Autodesk Inventor part; units mm, degrees
ref_plane "YZ Plane" through (0, 0, 0) normal (1, 0, 0) x (0, 1, 0)
ref_plane "XZ Plane" through (0, 0, 0) normal (0, 1, 0) x (-1, 0, 0)
ref_plane "XY Plane" through (0, 0, 0) normal (0, 0, 1) x (1, 0, 0)
sketch "Skizze1" plane through (0, 0, 0) normal (0, 1, 0) x (-1, 0, 0)
  line L0 (0, 0) -> (10, 0)
  line L1 (10, 0) -> (10, -30)
  line L2 (10, -30) -> (0, -30)
  line L3 (0, -30) -> (0, 0)
  dimension "d0" = 10
  dimension "d1" = 30
extrude "Extrusion1" add sketch "Skizze1" along normal blind 30
sketch "Skizze2" plane through (0, 30, 0) normal (0, 1, 0) x (1, 0, 0)
  line L0 (-10, 0) -> (0, 0)
  line L1 (0, 0) -> (0, 30)
  point P0 (-5, 4.75)
  point P1 (-5, 25.25)
  dimension "d4" = 20.5
  dimension "d5" = 4.75
  dimension "d6" = 5
hole "Bohrung1" at (-5, 30, -4.75) at (-5, 30, -25.25) direction (0, -1, 0) diameter 2 depth 10 tip angle 118
sketch "Skizze4" plane through (0, 0, 0) normal (0, -1, 0) x (1, 0, 0)
  line L0 (0, 0) -> (-10, 0)
  line L1 (0, -30) -> (0, 0)
  point P0 (-5, -22.5)
  point P1 (-5, -7.5)
  dimension "d21" = 15
  dimension "d22" = 7.5
  dimension "d23" = 5
hole "Bohrung3" at (-5, 0, -22.5) at (-5, 0, -7.5) direction (0, 1, 0) diameter 2.5 depth 10 tip angle 118
properties part number "KugelRadStützen"
Input: part model. Units: mm. Frame: model coordinates. A direction names the side the tool comes from. Give positions to 0.01 mm unless a question says otherwise; leave off trailing zeros. Order: outer loops, then holes, each group sorted by start corner. A loop starts at its lowest first (then second) coordinate and runs counter-clockwise, first axis right, second up.
1. Pin query (flat end, axial travel): pin 1 (1.5 mm diameter, centred on x = -5, z = -7.5, fed in from -Y). Return the tip coordinate at first contact, or that it passes through.
Derived:
pin 1: stops at y = 10.3
2. Material intervals for L1, parallel to X at y = 25, z = -4.75, sorted ascending.
Derived:
L1: x = -10 to -6, -4 to 0
3. Reachability of faces 4 (the flat face through (-5, 0, -15)), 5 (the cylindrical face through (-4.521, 5.07, -23.655)), 6 (the cylindrical face through (-5.676, 24.93, -25.987)) from +Z, -Z, +X, -X, +Y, -Y: full face, straight path, thin tool, end or side. Return the list, or none.
Derived:
face 4: +Z, -Z, +X, -X, -Y
face 5: -Y
face 6: +Y
4. Mould query, pull axis Z, two halves, no side actions, for faces 1 (the cylindrical face through (-4.24, 5.07, -6.51)), 2 (the flat face through (-5, 15, 0)), 3 (the flat face through (-5, 15, -30)). Classes: released by +Z, released by -Z, zero draft, split by the parting line, or undercut.
Derived:
face 1: undercut
face 2: released by +Z
face 3: released by -Z
5. Section B-B on y = 5. Return the cut outline in (x, z).
Derived:
outline: (-10, -30) - (0, -30) - (0, 0) - (-10, 0) - close; hole circle Ø2.5 at (-5, -22.5); hole circle Ø2.5 at (-5, -7.5)
6. Section A-A on y = 23.5. Return the cut outline in (x, z).
Derived:
outline: (-10, -30) - (0, -30) - (0, 0) - (-10, 0) - close; hole circle Ø2 at (-5, -25.25); hole circle Ø2 at (-5, -4.75)
